```python
from build123d import *

# Parameters (mm, degrees)
F0_W     = 100
F0_H     = 50
F1_DEPTH = 35
F2_R     = 6.25
F3_DEPTH = 50.001
F5_D     = 6
F6_R     = 10
F6_R_2   = 6.25
F7_DEPTH = 10


with BuildPart() as f1:
    # F0 (on Front) → F1 (new body)
    with BuildSketch(Plane.XZ):
        with Locations((50, 25)):
            Rectangle(F0_W, F0_H)
    extrude(amount=F1_DEPTH)

    # F2 (on face) → F3 (cut, through all)
    with BuildSketch(Plane.XY.offset(50)):
        with Locations((25, -17.5)):
            Circle(F2_R)
        with Locations((75, -17.5)):
            Circle(F2_R)
    extrude(amount=-F3_DEPTH, mode=Mode.SUBTRACT)

    # F5 (through all)
    with Locations(Plane(origin=(0, 0, 0), x_dir=(-1, 0, 0), z_dir=(0, 1, 0))):
        with Locations((-90, 40), (-10, 40), (-10, 10), (-90, 10)):
            Hole(F5_D / 2)

    # F6 (on face) → F7 (cut)
    with BuildSketch(Plane(origin=(0, 0, 0), x_dir=(1, 0, 0), z_dir=(0, 0, -1))):
        with Locations((25, 17.5)):
            Circle(F6_R)
        with Locations((25, 17.5)):
            Circle(F6_R_2, mode=Mode.SUBTRACT)
        with Locations((75, 17.5)):
            Circle(F6_R)
        with Locations((75, 17.5)):
            Circle(F6_R_2, mode=Mode.SUBTRACT)
    extrude(amount=-F7_DEPTH, mode=Mode.SUBTRACT)


solid = f1.part
```
Design review of the part built by this model. Coordinates are the model's own, in mm. A direction names the side the tool comes from. Give positions to 0.01 mm unless a question says otherwise; leave off trailing zeros. Write each loop counter-clockwise with the first axis right and the second up, starting at its lowest first coordinate (ties: lowest second). Pieces come first, ordered by that corner, then holes. Notation, with made-up numbers: (-6, 47.25) - (0, 47.25) arc R26 cw to (0, 70.25) - close; hole circle Ø7 at (70.25, 44). An arc over 180 degrees is marked (long way). Return JSON: item names as keys, results as strings. Group by question number.
(1) We need section C-C, the plane y = -33. Give the boundary of the cut face in (x, z).
(2) Insertion check: pin 1 (12 mm diameter, centred on x = 75, y = -17.5, fed in from -Z); pin 2 (6 mm diameter, centred on x = 70, y = -13, fed in from -Z). Each pin has a flat end and moves straight along its axis. Give the tip position at first contact, or say it passes through.
(3) Mouldability with a two-part tool opening along Y and no side actions: class faces 3 (the flat face through (49, 0, 25)), 4 (the cylindrical face through (34.54, -20.5, 4.93)), 5 (the flat face through (49, -35, 25)), 6 (the cylindrical face through (80.96, -15.62, 30.28)) as +Y half, -Y half, draft (parallel to the pull), parting line (faces both ways), or undercut.
(4) We need section B-B, the plane x = 75. Give the boundary of the cut face in (y, z), then the cut area to 3 significant figures.
(5) To check wall thickness, follow probe 1 along Z at (x, y) = (10, -11); probe 2 along X at (y, z) = (-27.5, 40.5); probe 3 along Z at (x, y) = (92, -4). State the ranges of each line that lie inside material, in increasing order.
(6) Machinability: for faces 1 (the cylindrical face through (20.39, -13.28, 30.28)), 2 (the flat face through (20, -13, 10)), which of the approach directions +Z, -Z, +X, -X, +Y, -Y give a long, thin tool a straight path to every point of the face, cutting with its end or side? Answer none if there is none.
(7) We need section A-A, the plane z = 40. Give the boundary of the cut face in (x, y), then the cut area to 3 significant figures.
(8) We need section D-D, the plane x = 90. Give the boundary of the cut face in (y, z).
Reported:
{
 "1": {"outline": "(0, 0) - (100, 0) - (100, 50) - (0, 50) - close; hole circle Ø6 at (10, 10); hole circle Ø6 at (10, 40); hole circle Ø6 at (90, 10); hole circle Ø6 at (90, 40)"},
 "2": {"pin 1": "passes through", "pin 2": "stops at z = 10"},
 "3": {"face 3": "+Y half", "face 4": "undercut", "face 5": "-Y half", "face 6": "undercut"},
 "4": {"outline": "(-35, 0) - (-27.5, 0) - (-27.5, 10) - (-23.75, 10) - (-23.75, 50) - (-35, 50) - close; (-11.25, 10) - (-7.5, 10) - (-7.5, 0) - (0, 0) - (0, 50) - (-11.25, 50) - close", "area": "1,050 mm2"},
 "5": {"probe 1": "z = 0 to 7, 13 to 37, 43 to 50", "probe 2": "x = 0 to 7.04, 12.96 to 87.04, 92.96 to 100", "probe 3": "z = 0 to 7.76, 12.24 to 37.76, 42.24 to 50"},
 "6": {"face 1": "+Z, -Z", "face 2": "-Z"},
 "7": {"outline": "(0, -35) - (7, -35) - (7, 0) - (0, 0) - close; (13, -35) - (87, -35) - (87, 0) - (13, 0) - close; (93, -35) - (100, -35) - (100, 0) - (93, 0) - close; hole circle Ø12.5 at (25, -17.5); hole circle Ø12.5 at (75, -17.5)", "area": "2,830 mm2"},
 "8": {"outline": "(-35, 0) - (0, 0) - (0, 7) - (-35, 7) - close; (-35, 13) - (0, 13) - (0, 37) - (-35, 37) - close; (-35, 43) - (0, 43) - (0, 50) - (-35, 50) - close"}
}
